Input: part model. Units: mm. Frame: model coordinates. A direction names the side the tool comes from. Give positions to 0.01 mm unless a question says otherwise; leave off trailing zeros. Loops run counter-clockwise (first coordinate to the right, second up) from the corner with the lowest first, then second, coordinate; pieces in that order, holes last. Notation, with made-up numbers: (74.5, 51.25) - (102.5, 51.25) arc R24 ccw to (102.5, 68.25) - close; hole circle Ø5 at (-2, 34.25). An arc over 180 degrees is marked (long way). Answer as a JSON object with one key per item and string values.
from build123d import *

# Parameters (mm, degrees)
SKETCH1_W           = 22
SKETCH1_H           = 11.5
BOSS_EXTRUDE1_DEPTH = 16.5
BOSS_EXTRUDE2_DEPTH = 2
SKETCH4_W           = 22
SKETCH4_H           = 11.5
BOSS_EXTRUDE3_DEPTH = 4
SKETCH5_R           = 5.5
BOSS_EXTRUDE4_DEPTH = 4
SKETCH7_R           = 3.5
BOSS_EXTRUDE5_DEPTH = 4


with BuildPart() as part:
    # Sketch1 → Boss-Extrude1 (new body)
    with BuildSketch(Plane(origin=(0, 0, 0), x_dir=(1, 0, 0), z_dir=(0, 1, 0))):
        Rectangle(SKETCH1_W, SKETCH1_H)
    extrude(amount=BOSS_EXTRUDE1_DEPTH)

    # Sketch2 → Boss-Extrude2 (add)
    with BuildSketch(Plane(origin=(0, 16.5, 0), x_dir=(1, 0, 0), z_dir=(0, 1, 0))):
        with BuildLine():
            Line((-15.5, 5.75), (15.5, 5.75))
            Line((15.5, 5.75), (15.5, 0.916515139))
            ThreePointArc((15.5, 0.916515139), (12.7, 0), (15.5, -0.916515139))
            Line((15.5, -0.916515139), (15.5, -5.75))
            Line((15.5, -5.75), (-15.5, -5.75))
            Line((-15.5, -5.75), (-15.5, -0.916515139))
            ThreePointArc((-15.5, -0.916515139), (-12.7, 0), (-15.5, 0.916515139))
            Line((-15.5, 0.916515139), (-15.5, 5.75))
        make_face()
    extrude(amount=BOSS_EXTRUDE2_DEPTH)

    # Sketch4 → Boss-Extrude3 (add)
    with BuildSketch(Plane(origin=(0, 18.5, 0), x_dir=(1, 0, 0), z_dir=(0, 1, 0))):
        Rectangle(SKETCH4_W, SKETCH4_H)
    extrude(amount=BOSS_EXTRUDE3_DEPTH)

    # Sketch5 → Boss-Extrude4 (add)
    with BuildSketch(Plane(origin=(0, 22.5, 0), x_dir=(1, 0, 0), z_dir=(0, 1, 0))):
        with Locations((5.5, 0)):
            Circle(SKETCH5_R)
    extrude(amount=BOSS_EXTRUDE4_DEPTH)

    # Sketch7 → Boss-Extrude5 (add)
    with BuildSketch(Plane(origin=(0, 26.5, 0), x_dir=(1, 0, 0), z_dir=(0, 1, 0))):
        with Locations((5.5, 0)):
            Circle(SKETCH7_R)
    extrude(amount=BOSS_EXTRUDE5_DEPTH)


solid = part.part
Item 1: Cut plane D-D (x = -8). Return loops of the section in (y, z).
Geometry check:
{"outline": "(0, -5.75) - (22.5, -5.75) - (22.5, 5.75) - (0, 5.75) - close"}
Item 2: Contact query for flat-ended pins moving along their axis: P1, Ø2, axis at x = 11.5, y = 8, coming from the -Z side; P2, Ø4, axis at x = 14.25, z = 0, coming from the -Y side; P3, Ø4, axis at x = 11, z = 2, coming from the +Y side; P4, Ø3.5, axis at y = 7, z = -0.5, coming from the +X side. Output: stop coordinate, or through.
Geometry check:
{"P1": "stops at z = -5.75", "P2": "stops at y = 16.5", "P3": "stops at y = 26.5", "P4": "stops at x = 11"}
Item 3: Cut plane A-A (x = 14.25). Return loops of the section in (y, z).
Geometry check:
{"outline": "(16.5, -5.75) - (18.5, -5.75) - (18.5, -1.55) - (16.5, -1.55) - close; (16.5, 1.55) - (18.5, 1.55) - (18.5, 5.75) - (16.5, 5.75) - close"}
Item 4: Access query for faces 5 (the face through (8.84, 28.47, -1.05)), 6 (the face through (-11, 8, 0)), 7 (the face through (12, 18.5, 0)). Directions: +Z, -Z, +X, -X, +Y, -Y. A direction counts if a zero-diameter tool reaches every point of the face in a straight line with its end or side. Return the directions, or none.
Geometry check:
{"face 5": "+Y", "face 6": "+Z, -Z, -X, -Y", "face 7": "+Z, -Z, +X, +Y"}
Item 5: Cut plane C-C (x = 5.5). Return loops of the section in (y, z), then the cut area to 3 significant figures.
Geometry check:
{"outline": "(0, -5.75) - (22.5, -5.75) - (22.5, -5.5) - (26.5, -5.5) - (26.5, -3.5) - (30.5, -3.5) - (30.5, 3.5) - (26.5, 3.5) - (26.5, 5.5) - (22.5, 5.5) - (22.5, 5.75) - (0, 5.75) - close", "area": "331 mm2"}
Item 6: Mould query, pull axis Z, two halves, no side actions, for faces 1 (the face through (12.7, 17.49, -0.05)), 2 (the face through (0, 11, 5.75)), 3 (the face through (0, 11, -5.75)), 4 (the face through (0, 0, 0)). Classes: released by +Z, released by -Z, zero draft, split by the parting line, or undercut.
Geometry check:
{"face 1": "undercut", "face 2": "released by +Z", "face 3": "released by -Z", "face 4": "zero draft"}
Item 7: Cut plane B-B (y = 8). Return loops of the section in (x, z).
Geometry check:
{"outline": "(-11, -5.75) - (11, -5.75) - (11, 5.75) - (-11, 5.75) - close"}
Item 8: Material intervals for line 1 (Z direction, x = 14.25, y = 17.8); line 2 (Y direction, x = 13.5, z = 2.5); line 3 (Y direction, x = 0.5, z = 4), sorted ascending. Write a range as [from, to].
Geometry check:
{"line 1": "z = [-5.75, -1.55], [1.55, 5.75]", "line 2": "y = [16.5, 18.5]", "line 3": "y = [0, 22.5]"}
